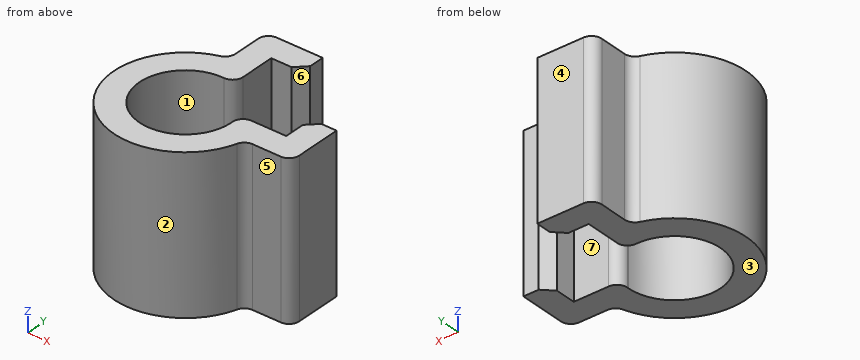
from build123d import *

# Parameters (mm, degrees)
F1_DEPTH = 15
F2_SIZE  = 1
F3_R     = 1


with BuildPart() as f1:
    # F0 (on Top) → F1 (new body)
    with BuildSketch(Plane.XY):
        with BuildLine():
            ThreePointArc((-2.5, 5.706772), (-1.251394, 5.834777), (0, 5.737742))
            Line((0, 5.737742), (0, 7.75))
            Line((0, 7.75), (3, 7.75))
            Line((3, 7.75), (3, 10.25))
            Line((3, 10.25), (-2.5, 10.25))
            Line((-2.5, 10.25), (-2.5, 5.706772))
        make_face()
        with BuildLine():
            ThreePointArc((3.181981, 0), (3.296816, -0.577318), (3.335314, -1.164686))
            ThreePointArc((3.335314, -1.164686), (-4.734776, -3.904112), (0, 3.181981))
            Line((0, 3.181981), (0, 5.737742))
            ThreePointArc((0, 5.737742), (-1.251394, 5.834777), (-2.5, 5.706772))
            ThreePointArc((-2.5, 5.706772), (-6.114433, -6.114433), (5.706772, -2.5))
            ThreePointArc((5.706772, -2.5), (5.803105, -1.835429), (5.835314, -1.164686))
            ThreePointArc((5.835314, -1.164686), (5.810879, -0.580303), (5.737742, 0))
            Line((5.737742, 0), (3.181981, 0))
        make_face()
        with BuildLine():
            Line((7.75, 0), (5.737742, 0))
            ThreePointArc((5.737742, 0), (5.810879, -0.580303), (5.835314, -1.164686))
            ThreePointArc((5.835314, -1.164686), (5.803105, -1.835429), (5.706772, -2.5))
            Line((5.706772, -2.5), (10.25, -2.5))
            Line((10.25, -2.5), (10.25, 3))
            Line((10.25, 3), (7.75, 3))
            Line((7.75, 3), (7.75, 0))
        make_face()
    extrude(amount=F1_DEPTH)

    # F2
    f2_edges = [f1.edges().sort_by_distance(p)[0] for p in [
        (3, 7.75, 7.5),
        (7.75, 3, 7.5),
    ]]
    chamfer(f2_edges, length=F2_SIZE)

    # F3
    f3_edges = [f1.edges().sort_by_distance(p)[0] for p in [
        (10.25, -2.5, 7.5),
        (0, 3.181981, 7.5),
        (-2.5, 10.25, 7.5),
        (3.181981, 0, 7.5),
        (-2.5, 5.706772, 7.5),
        (5.706772, -2.5, 7.5),
    ]]
    fillet(f3_edges, radius=F3_R)


solid = f1.part
For this review, take the finished solid that the model builds, in its own axes (mm). Face numbers are marked on the shaded views. A direction names the side the tool comes from. Round coordinates to 2 decimals unless told otherwise and drop trailing zeros. Write each loop counter-clockwise with the first axis right and the second up, starting at its lowest first coordinate (ties: lowest second). Pieces come first, ordered by that corner, then holes. Notation, with made-up numbers: M 82,84 L 136,84 A27 ccw 136,122 Z; hole C -4.5,-27 d7. An arc over 180 degrees is marked long. Write item = value, one per line. Start each with the question number.
(1) We need section D-D (x = 7.25). Give the boundary of the cut face in (y, z), then the cut area to 3 significant figures.
(2) We need section B-B (x = 1.5). Give the boundary of the cut face in (y, z), then the cut area to 3 significant figures.
(3) Clearance check with flat-ended pins moving along their axes: pin 1 Ø3 at (x, z) = (7.5, 7.5) entering from +Y; pin 2 Ø3 at (x, z) = (-6, 2.5) entering from +Y; pin 3 Ø0.6 at (y, z) = (1, 5) entering from -X; pin 4 Ø1.5 at (x, y) = (-6, 7) entering from +Z. State where each tip first meets the part, or that it passes through.
(4) The part is to be moulded in two halves that separate along Y. For the marked faces 1, 2, 3 and 4, say which applies: +Y half, -Y half, draft (parallel to the pull), parting line (faces both ways), or undercut.
(5) For line 1 along X through (y, z) = (-3.75, 8.25); line 2 along Y through (x, z) = (-4.5, 6.25); line 3 along Y through (x, z) = (-3.25, 4.25), list the stretches that pass through material, from the lowest coordinate up.
(6) We need section C-C (z = 9). Give the boundary of the cut face in (x, y).
(7) We need section A-A (y = 0.5). Give the boundary of the cut face in (x, z), then the cut area to 3 significant figures.
(8) For the marked faces 5, 6 and 7, list the 3-axis set-ups (+Z, -Z, +X, -X, +Y, -Y) from which the entire face can be reached by the end or side of a thin tool; tool diameter is ignored.
Results found:
q1.outline = M -2.5,0 L 0,0 L 0,15 L -2.5,15 Z
q1.area = 37.5 mm²
q2.outline = M -7.64,0 L -4.79,0 L -4.79,15 L -7.64,15 Z; M 7.75,0 L 10.25,0 L 10.25,15 L 7.75,15 Z
q2.area = 80.2 mm²
q3.pin_1 = 3
q3.pin_2 = 4.99
q3.pin_3 = -7.91
q3.pin_4 = through
q4.face_1 = undercut
q4.face_2 = parting line
q4.face_3 = draft
q4.face_4 = +Y half
q5.line_1 = -7.67 to -4.85, 2.52 to 5.34
q5.line_2 = -7.32 to -4.19, 1.86 to 4.99
q5.line_3 = -7.85 to -5.15, 2.82 to 5.52
q6.outline = M -3.21,5.53 A7 ccw long 5.53,-3.21 A1 cw 6.49,-2.5 L 9.25,-2.5 A1 ccw 10.25,-1.5 L 10.25,3 L 8.75,3 L 7.75,2 L 7.75,0 L 4.33,0 A1 ccw 3.33,-1.03 A4.5 cw 3.34,-1.16 A4.5 cw long -1.03,3.33 A1 ccw 0,4.33 L 0,7.75 L 2,7.75 L 3,8.75 L 3,10.25 L -1.5,10.25 A1 ccw -2.5,9.25 L -2.5,6.49 A1 cw Z
q7.outline = M -7.96,0 L -5.35,0 L -5.35,15 L -7.96,15 Z; M 7.75,0 L 10.25,0 L 10.25,15 L 7.75,15 Z
q7.area = 76.8 mm²
q8.face_5 = +Z, -Z, +X, -Y
q8.face_6 = +Z, -Z, +X
q8.face_7 = +Z, -Z, +Y
